from build123d import *

# Parameters (mm, degrees)
F0_W     = 53
F0_H     = 53.000004
F1_DEPTH = 10
F2_W     = 53
F2_H     = 53.000004
F2_W_2   = 51
F2_H_2   = 51.000002
F3_DEPTH = 1
F4_W     = 51
F4_H     = 51.000002
F5_DEPTH = 9


with BuildPart() as f1:
    # F0 (on Top) → F1 (new body)
    with BuildSketch(Plane.XY):
        Rectangle(F0_W, F0_H)
    extrude(amount=F1_DEPTH)

    # F2 (on face) → F3 (join)
    with BuildSketch(Plane(origin=(0, 0, 0), x_dir=(1, 0, 0), z_dir=(0, 0, -1))):
        Rectangle(F2_W, F2_H)
        Rectangle(F2_W_2, F2_H_2, mode=Mode.SUBTRACT)
    extrude(amount=F3_DEPTH)

    # F4 (on face) → F5 (cut)
    with BuildSketch(Plane.XY.offset(10)):
        Rectangle(F4_W, F4_H)
    extrude(amount=-F5_DEPTH, mode=Mode.SUBTRACT)


solid = f1.part
Input: part model. Units: mm. Frame: model coordinates. A direction names the side the tool comes from. Round coordinates to 2 decimals unless told otherwise and drop trailing zeros. Write each loop counter-clockwise with the first axis right and the second up, starting at its lowest first coordinate (ties: lowest second). Pieces come first, ordered by that corner, then holes.
1) Contact query for a flat-ended pin moving along its axis: P1, Ø3, axis at x = -17.5, y = 2, coming from the -Z side. Output: stop coordinate, or through.
2) Draft query along Y for faces 4 (the flat face through (0, -25.5, 6)), 5 (the flat face through (26.5, 0, 5)), 6 (the flat face through (0, 26.5, 5)). Return one class per face: pulls with the +Y half, pulls with the -Y half, needs draft (parallel to the pull), parting line crosses it, or undercut.
3) Ray query, L1, parallel to X at y = -3, z = 7; L2, parallel to Z at x = 1, y = 14. Return the intervals inside material, ascending.
4) Cut plane B-B (y = 5). Return the cut outline in (x, z).
5) Cut plane A-A (z = 8.75). Return the cut outline in (x, y), then the cut area to 3 significant figures.
6) Reachability of faces 1 (the flat face through (-26.5, 0, 5)), 2 (the flat face through (25.5, 0, 6)), 3 (the flat face through (0, 0, 0)) from +Z, -Z, +X, -X, +Y, -Y: full face, straight path, thin tool, end or side. Return the list, or none.
Geometry says:
1. P1: stops at z = 0
2. face 4: undercut
2. face 5: needs draft
2. face 6: pulls with the +Y half
3. L1: x = -26.5 to -25.5, 25.5 to 26.5
3. L2: z = 0 to 1
4. outline: (-26.5, -1) - (-25.5, -1) - (-25.5, 0) - (25.5, 0) - (25.5, -1) - (26.5, -1) - (26.5, 10) - (25.5, 10) - (25.5, 1) - (-25.5, 1) - (-25.5, 10) - (-26.5, 10) - close
5. outline: (-26.5, -26.5) - (26.5, -26.5) - (26.5, 26.5) - (-26.5, 26.5) - close; hole (-25.5, -25.5) - (25.5, -25.5) - (25.5, 25.5) - (-25.5, 25.5) - close
5. area: 208 mm2
6. face 1: +Z, -Z, -X, +Y, -Y
6. face 2: +Z
6. face 3: -Z
